Geometry check sheet. Reference: the model listing, model coordinates, mm. A direction names the side the tool comes from. Round coordinates to 2 decimals unless told otherwise and drop trailing zeros. Loops run counter-clockwise (first coordinate to the right, second up) from the corner with the lowest first, then second, coordinate; pieces in that order, holes last. Notation, with made-up numbers: (9, 9) -> (52, 9) arc R11 cw to (52, 17) -> close; hole circle Ø4 at (55.5, -11.75). An arc over 180 degrees is marked (long way). Use one line per item in the form item = value.
from build123d import *

# Parameters (mm, degrees)
SKETCH_1_R          = 15
EXTRUDE_1_DEPTH     = 10
CUT_EXTRUDE_1_DEPTH = 10
SKETCH_5_R          = 2
CUT_EXTRUDE_2_DEPTH = 25.779023387
SKETCH_7_W          = 30.648506912
SKETCH_7_H          = 10.688803122
CUT_EXTRUDE_4_DEPTH = 24.45207897
EXTRUDE_START       = -10
EXTRUDE_2_DEPTH     = 10
EXTRUDE_3_DEPTH     = 10
FILLET_1_R          = 2
FILLET_2_R          = 1


with BuildPart() as part:
    # ｽｹｯﾁ1 → ﾎﾞｽ - 押し出し1 (new body)
    with BuildSketch(Plane.XY):
        Circle(SKETCH_1_R)
    extrude(amount=EXTRUDE_1_DEPTH)

    # ｽｹｯﾁ2 → ｶｯﾄ - 押し出し1 (cut)
    with BuildSketch(Plane.XY.offset(10)):
        with BuildLine():
            Line((5.762811814, 2), (20.145888179, 2))
            Line((20.145888179, 2), (20.145888179, 26.748934653))
            Line((20.145888179, 26.748934653), (-19.854111821, 26.748934653))
            Line((-19.854111821, 26.748934653), (-19.854111821, 2))
            Line((-19.854111821, 2), (-5.762811814, 2))
            ThreePointArc((-5.762811814, 2), (0, -6.1), (5.762811814, 2))
        make_face()
    extrude(amount=-CUT_EXTRUDE_1_DEPTH, mode=Mode.SUBTRACT)

    # ｽｹｯﾁ5 → ｶｯﾄ - 押し出し2 (cut, through all)
    with BuildSketch(Plane(origin=(0, 2, 0), x_dir=(1, 0, 0), z_dir=(0, 1, 0))):
        with Locations(Location((-10.5, -5, 0), (0, 0, 270))):
            Circle(SKETCH_5_R)
        with Locations(Location((10.5, -5, 0), (0, 0, 270))):
            Circle(SKETCH_5_R)
    extrude(amount=-CUT_EXTRUDE_2_DEPTH, mode=Mode.SUBTRACT)

    # ｽｹｯﾁ7 → ｶｯﾄ - 押し出し4 (cut, through all)
    with BuildSketch(Plane.XY.offset(10)):
        with Locations((0, -13.344401561)):
            Rectangle(SKETCH_7_W, SKETCH_7_H)
    extrude(amount=-CUT_EXTRUDE_4_DEPTH, mode=Mode.SUBTRACT)

    # ｽｹｯﾁ8 → ﾎﾞｽ - 押し出し2 (add)
    with BuildSketch(Plane.XY.offset(10).offset(EXTRUDE_START)):
        with BuildLine():
            Line((-14.866068747, 2), (-15.5, 2))
            Line((-15.5, 2), (-15.5, -8))
            Line((-15.5, -8), (-12.68857754, -8))
            ThreePointArc((-12.68857754, -8), (-14.656555974, -3.191452176), (-14.866068747, 2))
        make_face()
        with BuildLine():
            ThreePointArc((14.866068747, 2), (14.656555974, -3.191452176), (12.68857754, -8))
            Line((12.68857754, -8), (15.5, -8))
            Line((15.5, -8), (15.5, 2))
            Line((15.5, 2), (14.866068747, 2))
        make_face()
    extrude(amount=EXTRUDE_2_DEPTH)

    # ｽｹｯﾁ9 → ﾎﾞｽ - 押し出し3 (add)
    with BuildSketch(Plane.XY.offset(10)):
        with BuildLine():
            Line((-6, -8), (6, -8))
            ThreePointArc((6, -8), (0, -10), (-6, -8))
        make_face()
    extrude(amount=-EXTRUDE_3_DEPTH)

    # ﾌｨﾚｯﾄ1
    fillet_1_edges = [part.edges().sort_by_distance(p)[0] for p in [
        (-15.5, -8, 5),
        (15.5, -8, 5),
    ]]
    fillet(fillet_1_edges, radius=FILLET_1_R)

    # ﾌｨﾚｯﾄ2
    fillet_2_edges = [part.edges().sort_by_distance(p)[0] for p in [
        (-15.5, 2, 5),
        (15.5, 2, 5),
    ]]
    fillet(fillet_2_edges, radius=FILLET_2_R)


solid = part.part
1. Section check B-B (z = 5). Record the boundary of the cut face in (x, y), then the cut area to 3 significant figures.
Return value:
outline = (-15.5, -6) arc R2 ccw to (-13.5, -8) -> (-12.5, -8) -> (-12.5, 2) -> (-14.5, 2) arc R1 ccw to (-15.5, 1) -> close; (-8.5, -8) -> (-6, -8) arc R10 ccw to (6, -8) -> (8.5, -8) -> (8.5, 2) -> (5.76, 2) arc R6.1 cw (long way) to (-5.76, 2) -> (-8.5, 2) -> close; (12.5, -8) -> (13.5, -8) arc R2 ccw to (15.5, -6) -> (15.5, 1) arc R1 ccw to (14.5, 2) -> (12.5, 2) -> close
area = 162 mm2
2. Gauge pin test, flat ends, axial feed: pin 1 (2 mm diameter, centred on x = -8.5, z = 6.5, fed in from -Y); pin 2 (1 mm diameter, centred on y = -7.5, z = 3.5, fed in from +X). Record the tip position at first contact, or that the pin passes through.
Return value:
pin_1 = -8
pin_2 = 15.23
3. Material ranges on line 1 along X through (y, z) = (-0.25, 5); line 2 along X through (y, z) = (0, 7.75); line 3 along X through (y, z) = (-7.75, 5.25), recorded low to high.
Return value:
line_1 = -15.5 to -12.5, -8.5 to -6.09, 6.09 to 8.5, 12.5 to 15.5
line_2 = -15.5 to -6.1, 6.1 to 15.5
line_3 = -14.47 to -12.48, -8.52 to 8.52, 12.48 to 14.47
4. Section check D-D (z = 2). Record the boundary of the cut face in (x, y), then the cut area to 3 significant figures.
Return value:
outline = (-15.5, -6) arc R2 ccw to (-13.5, -8) -> (-6, -8) arc R10 ccw to (6, -8) -> (13.5, -8) arc R2 ccw to (15.5, -6) -> (15.5, 1) arc R1 ccw to (14.5, 2) -> (5.76, 2) arc R6.1 cw (long way) to (-5.76, 2) -> (-14.5, 2) arc R1 ccw to (-15.5, 1) -> close
area = 242 mm2
5. Mould release check, pull along Z, two halves, no side actions. Record for faces 3 (the flat face through (8, -8, 5)), 4 (the flat face through (0, -7, 0)), 5 (the cylindrical face through (-9.148, -2.93, 3.526)): released by +Z, released by -Z, zero draft, split by the parting line, or undercut.
Return value:
face_3 = zero draft
face_4 = released by -Z
face_5 = undercut
6. Tool access check on faces 1 (the flat face through (-8, -8, 5)), 2 (the cylindrical face through (-0.163, -6.098, 5.07)). Record the directions out of +Z, -Z, +X, -X, +Y, -Y that give a thin tool (end or side, any length) a straight path to the whole face; none if there is none.
Return value:
face_1 = +Z, -Z, -X, -Y
face_2 = +Z, -Z
7. Section check C-C (y = -5.5). Record the boundary of the cut face in (x, z), then the cut area to 3 significant figures.
Return value:
outline = (-15.5, 0) -> (-2.64, 0) -> (-2.64, 10) -> (-15.5, 10) -> close; (2.64, 0) -> (15.5, 0) -> (15.5, 10) -> (2.64, 10) -> close; hole circle Ø4 at (-10.5, 5); hole circle Ø4 at (10.5, 5)
area = 232 mm2
8. Section check A-A (x = 10.5). Record the boundary of the cut face in (y, z).
Return value:
outline = (-8, 0) -> (2, 0) -> (2, 3) -> (-8, 3) -> close; (-8, 7) -> (2, 7) -> (2, 10) -> (-8, 10) -> close
